Work out the finished part from the listing and answer in its coordinate system (mm). A direction names the side the tool comes from. Coordinates: 2 decimals unless noted, no trailing zeros. Loops run counter-clockwise (first coordinate to the right, second up) from the corner with the lowest first, then second, coordinate; pieces in that order, holes last. Notation, with made-up numbers: (-5, -11.75) -> (18, -11.75) arc R18 cw to (18, 12.25) -> close; hole circle Ø5 at (83, -36). An arc over 180 degrees is marked (long way). Use a Markdown table: item, result.
from build123d import *

# Parameters (mm, degrees)
F0_W     = 3.048
F0_H     = 5.588
F1_DEPTH = 3.81


with BuildPart() as f1:
    # F0 (on Top) → F1 (new body)
    with BuildSketch(Plane.XY):
        with BuildLine():
            ThreePointArc((0, -25.4), (-16.51, 19.302329), (25.093028, -3.937))
            ThreePointArc((25.093028, -3.937), (27.737531, -7.565753), (31.366284, -4.92125))
            ThreePointArc((31.366284, -4.92125), (-20.169598, 24.520396), (-1.221154, -31.726508))
            ThreePointArc((-1.221154, -31.726508), (-0.354868, -32.114981), (0, -32.995568))
            Line((0, -32.995568), (0, -45.72))
            ThreePointArc((0, -45.72), (0.371974, -46.618026), (1.27, -46.99))
            Line((1.27, -46.99), (5.08, -46.99))
            ThreePointArc((5.08, -46.99), (5.978026, -46.618026), (6.35, -45.72))
            Line((6.35, -45.72), (6.35, -31.75))
            ThreePointArc((6.35, -31.75), (4.490128, -27.259872), (0, -25.4))
        make_face()
        with Locations((3.175, -39.37)):
            Rectangle(F0_W, F0_H, mode=Mode.SUBTRACT)
    extrude(amount=F1_DEPTH)


solid = f1.part
Q1. Determine the mould class of faces 4 (the flat face through (3, -46.99, 2)), 5 (the flat face through (4.699, -39, 2)), 6 (the flat face through (0, -39, 2)), 7 (the flat face through (1.651, -39, 2)) for opening direction Y: pulls with the +Y half, pulls with the -Y half, needs draft (parallel to the pull), parting line crosses it, or undercut.
Solved:
| item | result |
|---|---|
| face 4 | pulls with the -Y half |
| face 5 | undercut |
| face 6 | needs draft |
| face 7 | undercut |
Q2. Section C-C on x = -14 is taken. Determine the outline of the cut face in (y, z).
Solved:
| item | result |
|---|---|
| outline | (-28.5, 0) -> (-21.19, 0) -> (-21.19, 3.81) -> (-28.5, 3.81) -> close; (21.19, 0) -> (28.5, 0) -> (28.5, 3.81) -> (21.19, 3.81) -> close |
Q3. Section D-D on x = 13 is taken. Determine the outline of the cut face in (y, z), and give its area (3 significant figures).
Solved:
| item | result |
|---|---|
| outline | (21.82, 0) -> (28.97, 0) -> (28.97, 3.81) -> (21.82, 3.81) -> close |
| area | 27.2 mm² |
Q4. For faces 1 (the flat face through (6.35, -39, 2)), 2 (the flat face through (3, -42.164, 2)), 3 (the cylindrical face through (4.54, -27.31, 1.88)), determine the directions among +Z, -Z, +X, -X, +Y, -Y from which every point of the face is accessible in a straight line to the end or side of a thin tool.
Solved:
| item | result |
|---|---|
| face 1 | +Z, -Z, +X, -Y |
| face 2 | +Z, -Z |
| face 3 | +Z, -Z, +X |
Q5. Consider line 1 (X direction, y = 0, z = 2.9); line 2 (X direction, y = -5, z = 2.1); line 3 (Y direction, x = -18.5, z = 1.55). Determine where each line is inside the solid, lowest interval first. Write a range as [from, to].
Solved:
| item | result |
|---|---|
| line 1 | [-31.75, -25.4], [25.4, 31.75] |
| line 2 | [-31.35, -24.9], [25.11, 31.35] |
| line 3 | [-25.8, -17.4], [17.4, 25.8] |
Q6. Given pin 1 Ø0.9 at (x, z) = (2.5, 2) entering from +Y; pin 2 Ø1.5 at (x, z) = (18, 2.5) entering from -Y; pin 3 Ø1.9 at (y, z) = (-39.5, 2) entering from +X; pin 4 Ø10 at (x, y) = (-23, -32) entering from +Z, each flat-ended and moving along its own axis, determine where each tip first touches the part or whether it passes through.
Solved:
| item | result |
|---|---|
| pin 1 | y = 31.68 |
| pin 2 | y = 17.13 |
| pin 3 | x = 6.35 |
| pin 4 | through |
Q7. Section A-A on y = 0 is taken. Determine the outline of the cut face in (x, z).
Solved:
| item | result |
|---|---|
| outline | (-31.75, 0) -> (-25.4, 0) -> (-25.4, 3.81) -> (-31.75, 3.81) -> close; (25.4, 0) -> (31.75, 0) -> (31.75, 3.81) -> (25.4, 3.81) -> close |
